Check sheet for the modelled part. Datum: model origin and axes. Units: mm. Face numbers are marked on the shaded views. A direction names the side the tool comes from. Give positions to 0.01 mm unless a question says otherwise; leave off trailing zeros. Order: outer loops, then holes, each group sorted by start corner. A loop starts at its lowest first (then second) coordinate and runs counter-clockwise, first axis right, second up. Notation, with made-up numbers: M 35.25,54 L 89.25,54 A33 cw 89.25,83 Z; hole C 45,33.5 d3. An arc over 180 degrees is marked long. One line per question, with ' | ' between items. Start each with the question number.
Autodesk Inventor part; units mm, degrees
ref_plane "YZ Plane" through (0, 0, 0) normal (1, 0, 0) x (0, 1, 0)
ref_plane "XZ Plane" through (0, 0, 0) normal (0, 1, 0) x (-1, 0, 0)
ref_plane "XY Plane" through (0, 0, 0) normal (0, 0, 1) x (1, 0, 0)
sketch "Sketch1" plane through (0, 0, 0) normal (0, 0, 1) x (1, 0, 0)
  circle A0 centre (1.2, 90) radius 1.7
  circle A1 centre (1.2, 90) radius 5
  point P0 (0, 0)
  dimension "d0" = 10
extrude "Extrusion1" add sketch "Sketch1" along normal blind 4.5
sketch "Sketch2" plane through (1.2, 90, 4.5) normal (0, 0, 1) x (1, 0, 0)
  circle A0 centre (0, 0) radius 1.7
  line L0 (31, 14.6742) -> (31, -15.3258) construction
  circle A1 centre (0, 0) radius 5
  line L1 (31, 14.6742) -> (31, 18.6742)
  line L2 (31, 18.6742) -> (0, 5)
  line L3 (31, -15.3258) -> (31, -19.3258)
  line L4 (31, -19.3258) -> (0, -5)
  line L5 (31, 14.6742) -> (4.5193, 2.1392)
  line L6 (31, -15.3258) -> (4.4822, -2.2159)
  arc A2 (0, 5) -> (0, -5) centre (0, 0) ccw
  arc A3 (4.4822, -2.2159) -> (4.5193, 2.1392) centre (0, 0) ccw
  point P0 (-1.2, -90)
  dimension "d3" = 31
  dimension "d4" = 30
  dimension "d5" = 4
  dimension "d6" = 4
extrude "Extrusion2" add sketch "Sketch2" along normal blind 3 contours A0 | A1 | A1 L2 L1 L5 | L6 L3 L4 A1
sketch "Sketch3" plane through (1.2, 90, 7.5) normal (0, 0, 1) x (1, 0, 0)
  circle A0 centre (0, 0) radius 1.7
  point P0 (-1.2, -90)
hole "Hole1" at (1.2, 90, 7.5) direction (0, 0, -1) diameter 3.4 end through all counterbore diameter 6.2 counterbore depth 2
sketch "Sketch4" plane through (1.2, 90, 7.5) normal (0, 0, 1) x (1, 0, 0)
  line L0 (31, 18.6742) -> (0, 5)
  line L1 (31, 18.6742) -> (29, 18.6742)
  line L2 (29, 18.6742) -> (29, 14.6742)
  line L3 (29, 14.6742) -> (31, 14.6742)
  line L4 (31, 14.6742) -> (31, 18.6742)
  line L5 (31, -19.3258) -> (31, -15.3258)
  line L6 (31, -15.3258) -> (29, -15.3258)
  line L7 (29, -15.3258) -> (29, -19.3258)
  line L8 (29, -19.3258) -> (31, -19.3258)
  line L9 (31, -19.3258) -> (31, -15.3258)
  point P0 (-1.2, -90)
  dimension "d16" = 2
  dimension "d17" = 2
extrude "Extrusion3" add sketch "Sketch4" along normal blind 14
sketch "Sketch5" plane through (30.2, 107.792, 7.5) normal (-1, 0, 0) x (0, 0, 1)
  line L0 (0, 0.8822) -> (14, 0.8822)
  line L1 (0, -3.1178) -> (14, -3.1178)
  line L2 (14, 0.8822) -> (12, 0.8822)
  line L3 (12, 0.8822) -> (12, -3.1178)
  line L4 (12, -3.1178) -> (14, -3.1178)
  line L5 (14, -3.1178) -> (14, 0.8822)
  line L6 (0, -33.1178) -> (14, -33.1178)
  line L7 (0, -37.1178) -> (14, -37.1178)
  line L8 (14, -33.1178) -> (12, -33.1178)
  line L9 (12, -33.1178) -> (12, -37.1178)
  line L10 (12, -37.1178) -> (14, -37.1178)
  line L11 (14, -37.1178) -> (14, -33.1178)
  point P0 (-7.5, -107.792)
  dimension "d20" = 2
extrude "Extrusion4" add sketch "Sketch5" along normal blind 4
properties part number "microphone_fix"
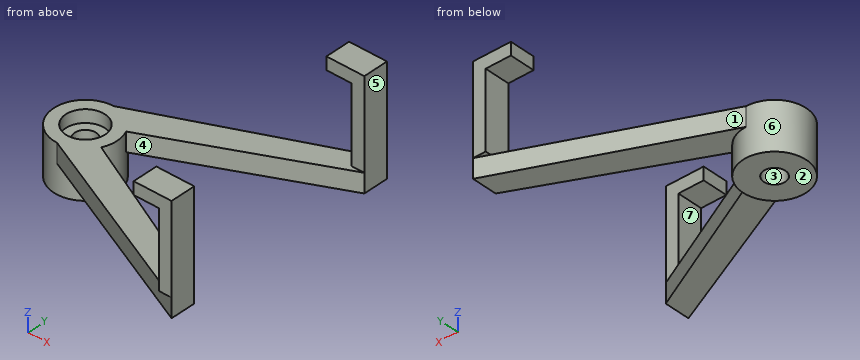
Item 1: Section check A-A, the plane z = 16.5. Record the cut outline in (x, y), then the cut area to 3 significant figures.
Item 2: Draft check along Y on the marked faces 1, 2, 3 and 4. Enter one of: released by +Y, released by -Y, zero draft, split by the parting line, or undercut.
Item 3: Scan lines: probe 1 along Y at (x, z) = (1.2, 6.85); probe 2 along Y at (x, z) = (1.2, 2.15); probe 3 along Z at (x, y) = (6.5, 84). Record each from-to range of solid material in increasing order. Write a range as [from, to].
Item 4: Section check C-C, the plane y = 106.5. Record the cut outline in (x, z), then the cut area to 3 significant figures.
Item 5: Set-up check for the marked faces 5, 6 and 7: record each of +Z, -Z, +X, -X, +Y, -Y from which the full face is reachable in a straight line by a thin tool's end or side.
Item 6: Go/stop test with flat-tipped pins: P1, Ø4.5, axis at x = 1.2, y = 90, coming from the +Z side; P2, Ø2, axis at y = 72.5, z = 15, coming from the -X side; P3, Ø4, axis at x = 26.5, z = 4.5, coming from the -Y side. Record where each tip stops, or that it passes through.
Item 7: Section check B-B, the plane x = 23. Record the cut outline in (y, z).
Item 8: Section check D-D, the plane y = 73. Record the cut outline in (x, z).
Reported:
1) outline: M 30.2,70.67 L 32.2,70.67 L 32.2,74.67 L 30.2,74.67 Z; M 30.2,104.67 L 32.2,104.67 L 32.2,108.67 L 30.2,108.67 Z | area: 16.0 mm^2
2) face 1: released by +Y | face 2: zero draft | face 3: undercut | face 4: undercut
3) probe 1: y = [85, 86.9], [93.1, 95] | probe 2: y = [85, 88.3], [91.7, 95] | probe 3: z = [4.5, 7.5]
4) outline: M 26.2,19.5 L 30.2,19.5 L 30.2,7.5 L 27.27,7.5 L 27.27,4.5 L 32.2,4.5 L 32.2,21.5 L 26.2,21.5 Z | area: 50.8 mm^2
5) face 5: +Z, -Z, +X, +Y, -Y | face 6: -Z | face 7: -X, +Y, -Y
6) P1: stops at z = 5.5 | P2: stops at x = 30.2 | P3: stops at y = 72.38
7) outline: M 74.93,4.5 L 79.22,4.5 L 79.22,7.5 L 74.93,7.5 Z; M 100.32,4.5 L 104.62,4.5 L 104.62,7.5 L 100.32,7.5 Z
8) outline: M 26.2,19.5 L 30.2,19.5 L 30.2,7.5 L 27.17,7.5 L 27.17,4.5 L 32.2,4.5 L 32.2,21.5 L 26.2,21.5 Z
